The model under review builds one solid part; all positions refer to its coordinate system, in mm. A direction names the side the tool comes from. Coordinates: 2 decimals unless noted, no trailing zeros. Order: outer loops, then holes, each group sorted by start corner. A loop starts at its lowest first (then second) coordinate and runs counter-clockwise, first axis right, second up. Notation, with made-up numbers: M 89,-25.5 L 98,-25.5 A20 cw 98,-6.5 Z; hole C 89.5,72 d6. An arc over 180 degrees is marked long. Answer as CSV lines item,"result". Start each with the question number.
Q1. The part is to be moulded in two halves that separate along X. For faces 1 (the face through (4.9, 5.4, 24.3)), 2 (the face through (5, 4, 21)), 3 (the face through (-4.9, 5.4, 24.3)), 4 (the face through (-2.5, 2, 17)), say which applies: +X half, -X half, draft (parallel to the pull), parting line (faces both ways), or undercut.
Q2. For P1, Ø1.5, axis at x = -3.5, y = 4.5, coming from the -Z side; P2, Ø8, axis at x = -5.5, z = 9, coming from the +Y side; P3, Ø4.5, axis at y = 1, z = 17, coming from the -X side; P4, Ø1, axis at y = 5, z = 13.5, coming from the -X side, all flat-tipped, find the tip position at first contact; note any pin that passes through.
Q3. Wall thickness on L1, parallel to Z at x = 0, y = 1.35; L2, parallel to X at y = 1.8, z = 0; L3, parallel to Z at x = -3.5, y = 2.5: over which ranges is each line inside the solid? List them lowest first. Write a range as [from, to].
Q4. Machinability: for faces 5 (the face through (1, 4, 8)), 6 (the face through (2.5, 2, 17)), 7 (the face through (-3.32, 1.97, 8.99)), 8 (the face through (0, 2, -8)), which of the approach directions +Z, -Z, +X, -X, +Y, -Y give a long, thin tool a straight path to every point of the face, cutting with its end or side? Answer none if there is none.
Q5. Consider section D-D on y = 2.25. Write out the cut boundary in (x, z), and give its area (3 significant figures).
Q6. Consider section C-C on y = 6.75. Write out the cut boundary in (x, z), and give its area (3 significant figures).
Q7. Consider section A-A on z = 23.5. Write out the cut boundary in (x, y), and give its area (3 significant figures).
Q8. Consider section B-B on x = 0. Write out the cut boundary in (y, z), and give its area (3 significant figures).
from build123d import *

# Parameters (mm, degrees)
SKETCH1_R           = 6
SKETCH1_R_2         = 1.1
BOSS_EXTRUDE1_DEPTH = 4
BOSS_EXTRUDE2_DEPTH = 6.5


with BuildPart() as part:
    # Sketch1 → Boss-Extrude1 (new body)
    with BuildSketch(Plane(origin=(0, 0, 0), x_dir=(1, 0, 0), z_dir=(0, 1, 0))):
        with BuildLine():
            Line((-2.5, -27.5), (2.5, -27.5))
            Line((2.5, -27.5), (2.5, -12.951833847))
            ThreePointArc((2.5, -12.951833847), (3.295532486, -9.043154047), (5.555555556, -5.756370599))
            ThreePointArc((5.555555556, -5.756370599), (0, 8), (-5.555555556, -5.756370599))
            ThreePointArc((-5.555555556, -5.756370599), (-3.295532486, -9.043154047), (-2.5, -12.951833847))
            Line((-2.5, -12.951833847), (-2.5, -27.5))
        make_face()
        Circle(SKETCH1_R, mode=Mode.SUBTRACT)
        with Locations((0, -23.5)):
            Circle(SKETCH1_R_2, mode=Mode.SUBTRACT)
    extrude(amount=BOSS_EXTRUDE1_DEPTH)

    # Sketch2 → Boss-Extrude2 (add)
    with BuildSketch(Plane.XY.offset(27.5)):
        with BuildLine():
            Line((-1.997835367, 4), (-2.5, 0))
            ThreePointArc((-2.5, 0), (-6.135441291, 3.080743774), (-7, 7.766888651))
            ThreePointArc((-7, 7.766888651), (-4.877255668, 5.381037947), (-1.997835367, 4))
        make_face()
    boss_extrude2 = extrude(amount=-BOSS_EXTRUDE2_DEPTH)

    # Mirror1: Boss-Extrude2 across plane
    add(boss_extrude2.mirror(Plane(origin=(0, 0, 0), x_dir=(0, 0, 1), z_dir=(1, 0, 0))))


solid = part.part
Evaluation:
1,face 1,"undercut"
1,face 2,"draft"
1,face 3,"undercut"
1,face 4,"-X half"
2,P1,"stops at z = -7.44"
2,P2,"stops at y = 4"
2,P3,"stops at x = -2.5"
2,P4,"passes through"
3,L1,"z = [-8, -6], [6, 22.4], [24.6, 27.5]"
3,L2,"x = [-8, -6], [6, 8]"
3,L3,"z = [-7.19, -4.87], [4.87, 8.59], [21, 27.5]"
4,face 5,"-Z, +Y"
4,face 6,"+X, +Y, -Y"
4,face 7,"-X, +Y, -Y"
4,face 8,"+Y, -Y"
5,outline,"M -5.57,21 L -2.5,21 L -2.5,12.95 A10 cw -5.56,5.76 A8 ccw long 5.56,5.76 A10 cw 2.5,12.95 L 2.5,21 L 5.57,21 L 5.57,27.5 L -5.57,27.5 Z; hole C 0,0 d12; hole C 0,23.5 d2.2"
5,area,"229 mm²"
6,outline,"M -7.09,21 L -6.3,21 L -6.3,27.5 L -7.09,27.5 Z; M 6.3,21 L 7.09,21 L 7.09,27.5 L 6.3,27.5 Z"
6,area,"10.3 mm²"
7,outline,"M -7,7.77 A7.09 ccw -2.5,0 L -1.1,0 L -1.1,4 L -2,4 A8.11 cw Z; M 1.1,0 L 2.5,0 A7.09 ccw 7,7.77 A8.11 cw 2,4 L 1.1,4 Z"
7,area,"45.4 mm²"
8,outline,"M 0,-8 L 4,-8 L 4,-6 L 0,-6 Z; M 0,6 L 4,6 L 4,22.4 L 0,22.4 Z; M 0,24.6 L 4,24.6 L 4,27.5 L 0,27.5 Z"
8,area,"85.2 mm²"
